Drawing for the job (mm, zero at the part's lowest x, y, z). A direction names the side the tool comes from. Round coordinates to 2 decimals unless told otherwise and drop trailing zeros. Write each loop counter-clockwise with the first axis right and the second up, starting at its lowest first coordinate (ties: lowest second). Pieces come first, ordered by that corner, then holes.
Item 1: 3-axis set-ups, long thin cutter, end or side, ignore diameter. For the marked faces 1 and 2: which of +Z, -Z, +X, -X, +Y, -Y reach the whole face in a straight line?
Item 2: Band-saw the part on D-D, the plane z = 34. Write the cut outline in (x, y), then the cut area to 3 significant figures.
Item 3: Band-saw the part on B-B, the plane x = 12.7. Write the cut outline in (y, z), then the cut area to 3 significant figures.
Item 4: Band-saw the part on C-C, the plane z = 25.4. Write the cut outline in (x, y).
Item 5: Drop flat-ended pins along their axis: pin 1 Ø12.5 at (x, y) = (18, 33) entering from +Z; pin 2 Ø2 at (x, z) = (22.225, 34.925) entering from -Y; pin 3 Ø1.5 at (x, z) = (9.5, 34) entering from +Y. Give the stop position or say it passes through.
Item 6: Mould opens along X. For the marked faces 3, 4 and 5 say: +X half, -X half, draft (parallel to the pull), parting line (faces both ways), or undercut.
Item 7: Band-saw the part on A-A, the plane y = 26.67. Write the cut outline in (x, z), then the cut area to 3 significant figures.
Item 8: Wall check: probe 1 along Y at (x, z) = (12.7, 2.5); probe 2 along X at (y, z) = (3.25, 44.45); probe 3 along Y at (x, z) = (21.5, 43.5). Give the ranges that are in metal, low to high.
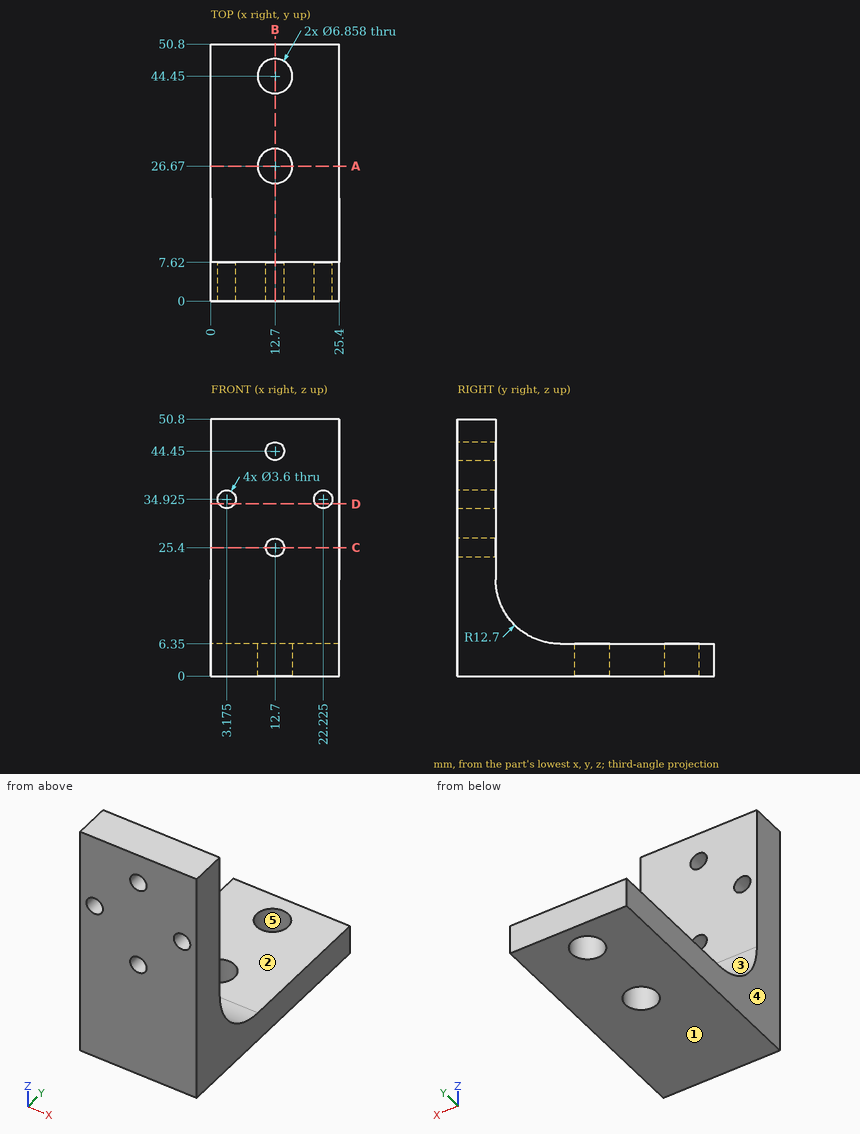
Results:
1. face 1: -Z, +X, -X, +Y, -Y
1. face 2: +Z, +X, -X, +Y
2. outline: (0, 0) - (1.63, 0) - (1.63, 7.62) - (0, 7.62) - close; (4.72, 0) - (20.68, 0) - (20.68, 7.62) - (4.72, 7.62) - close; (23.77, 0) - (25.4, 0) - (25.4, 7.62) - (23.77, 7.62) - close
2. area: 146 mm2
3. outline: (0, 0) - (23.24, 0) - (23.24, 6.35) - (20.32, 6.35) arc R12.7 cw to (7.62, 19.05) - (7.62, 23.6) - (0, 23.6) - close; (0, 27.2) - (7.62, 27.2) - (7.62, 42.65) - (0, 42.65) - close; (0, 46.25) - (7.62, 46.25) - (7.62, 50.8) - (0, 50.8) - close; (30.1, 0) - (41.02, 0) - (41.02, 6.35) - (30.1, 6.35) - close; (47.88, 0) - (50.8, 0) - (50.8, 6.35) - (47.88, 6.35) - close
3. area: 554 mm2
4. outline: (0, 0) - (10.9, 0) - (10.9, 7.62) - (0, 7.62) - close; (14.5, 0) - (25.4, 0) - (25.4, 7.62) - (14.5, 7.62) - close
5. pin 1: stops at z = 6.35
5. pin 2: passes through
5. pin 3: stops at y = 7.62
6. face 3: draft
6. face 4: -X half
6. face 5: undercut
7. outline: (0, 0) - (9.27, 0) - (9.27, 6.35) - (0, 6.35) - close; (16.13, 0) - (25.4, 0) - (25.4, 6.35) - (16.13, 6.35) - close
7. area: 118 mm2
8. probe 1: y = 0 to 23.24, 30.1 to 41.02, 47.88 to 50.8
8. probe 2: x = 0 to 10.9, 14.5 to 25.4
8. probe 3: y = 0 to 7.62
